The listing builds one solid part. Answer for the finished solid, in the listing's coordinates (mm). Face numbers are marked on the shaded views. A direction names the side the tool comes from. Coordinates: 2 decimals unless noted, no trailing zeros. Loops run counter-clockwise (first coordinate to the right, second up) from the corner with the lowest first, then second, coordinate; pieces in that order, holes last. Notation, with made-up numbers: (1.25, 14.5) -> (29.25, 14.5) arc R16 cw to (29.25, 32.5) -> close; hole circle Ø8 at (-12, 1). An arc over 180 degrees is marked (long way). Answer in a Markdown table with one row per item.
```python
from build123d import *

# Parameters (mm, degrees)
BOSS_EXTRUDE1_DEPTH = 34
SKETCH2_W           = 6.25
SKETCH2_H           = 31.7
CUT_EXTRUDE1_DEPTH  = 12
SKETCH3_W           = 10
SKETCH3_H           = 25
CUT_EXTRUDE2_DEPTH  = 12
SKETCH4_W           = 6
SKETCH4_H           = 10
CUT_EXTRUDE3_DEPTH  = 10
CHAMFER2_SIZE       = 1.5
CHAMFER3_SIZE       = 1.5
CHAMFER4_SIZE       = 1.5
CHAMFER4_SIZE_2     = 4.815472512


with BuildPart() as part:
    # Sketch1 → Boss-Extrude1 (new body)
    with BuildSketch(Plane(origin=(0, 0, 0), x_dir=(1, 0, 0), z_dir=(0, 1, 0))):
        Polygon((6.5, 4.75), (12.5, 4.75), (6.5, -4.75), (-6.5, -4.75), (-6.5, 4.75), align=None)
    extrude(amount=BOSS_EXTRUDE1_DEPTH)

    # Sketch2 → Cut-Extrude1 (cut)
    with BuildSketch(Plane.ZY.offset(6.5)):
        with Locations((0, 17)):
            Rectangle(SKETCH2_W, SKETCH2_H)
    extrude(amount=-CUT_EXTRUDE1_DEPTH, mode=Mode.SUBTRACT)

    # Sketch3 → Cut-Extrude2 (cut)
    with BuildSketch(Plane.XY.offset(4.75)):
        with Locations((-1.5, 17)):
            Rectangle(SKETCH3_W, SKETCH3_H)
    extrude(amount=-CUT_EXTRUDE2_DEPTH, mode=Mode.SUBTRACT)

    # Sketch4 → Cut-Extrude3 (cut)
    with BuildSketch(Plane.XY.offset(4.75)):
        with Locations((9.5, 29)):
            Rectangle(SKETCH4_W, SKETCH4_H)
        with Locations((9.5, 5)):
            Rectangle(SKETCH4_W, SKETCH4_H)
    extrude(amount=-CUT_EXTRUDE3_DEPTH, mode=Mode.SUBTRACT)

    # Chamfer2
    chamfer2_edges = [part.edges().sort_by_distance(p)[0] for p in [
        (6.5, 29, 4.75),
    ]]
    chamfer(chamfer2_edges, length=CHAMFER2_SIZE)

    # Chamfer3
    chamfer3_edges = [part.edges().sort_by_distance(p)[0] for p in [
        (6.5, 5, 4.75),
    ]]
    chamfer(chamfer3_edges, length=CHAMFER3_SIZE)

    # Chamfer4
    # the kernel refuses this chamfer: 4.815472512, 1.5 mm, written as the material it takes off along each edge
    with BuildSketch(Plane(origin=(6.5, -2.508851902, 4.75), x_dir=(-0.9965532165776719, 0, 0.08295593124482357), z_dir=(0, 1, 0))) as chamfer4_piece_1:
        Polygon((CHAMFER4_SIZE * 0.996553216578, -CHAMFER4_SIZE * 0.0829559312448), (-CHAMFER4_SIZE_2 * 0.602290752459, -CHAMFER4_SIZE_2 * 0.798276799955), (0, 0), align=None)
    extrude(amount=39.017703804, mode=Mode.SUBTRACT)


solid = part.part
```
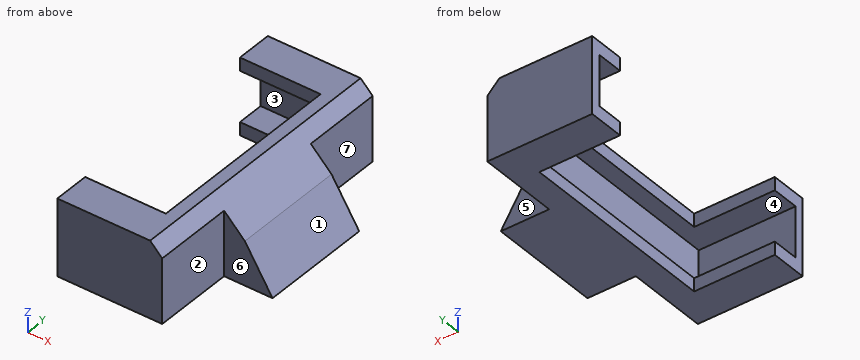
Item 1: Find the intervals of material crossed by probe 1 along Y at (x, z) = (0.75, -1.25); probe 2 along Z at (x, y) = (0.25, 31) (3 decimals); probe 3 along X at (y, z) = (9, 0.5), in increasing order.
Findings below:
| item | result |
|---|---|
| probe 1 | y = 0 to 1.15, 32.85 to 34 |
| probe 2 | z = -4.75 to -3.125, 3.125 to 4.75 |
| probe 3 | x = 5.5 to 6.5 |
Item 2: A cutting plane is placed at B-B, the plane y = 8. Determine the outline of the cut face in (x, z) (3 decimals), plus the area to 3 significant figures.
Findings below:
| item | result |
|---|---|
| outline | (3.5, -4.75) -> (6.5, -4.75) -> (6.5, 3.25) -> (5, 4.75) -> (3.5, 4.75) -> (3.5, 3.125) -> (5.5, 3.125) -> (5.5, -3.125) -> (3.5, -3.125) -> close |
| area | 14.9 mm2 |
Item 3: A tool of negligible diameter and unlimited length cuts with its end or side. For the marked faces 1, 2 and 3, from which of +Z, -Z, +X, -X, +Y, -Y can it reach the whole face along a straight path? Write none if from no direction.
Findings below:
| item | result |
|---|---|
| face 1 | +Z, +X, +Y, -Y |
| face 2 | +Z, -Z, +X, -Y |
| face 3 | -X |
Item 4: A cutting plane is placed at D-D, the plane x = 0.25. Determine the outline of the cut face in (y, z) (3 decimals), plus the area to 3 significant figures.
Findings below:
| item | result |
|---|---|
| outline | (0, -4.75) -> (4.5, -4.75) -> (4.5, -3.125) -> (1.15, -3.125) -> (1.15, 3.125) -> (4.5, 3.125) -> (4.5, 4.75) -> (0, 4.75) -> close; (29.5, -4.75) -> (34, -4.75) -> (34, 4.75) -> (29.5, 4.75) -> (29.5, 3.125) -> (32.85, 3.125) -> (32.85, -3.125) -> (29.5, -3.125) -> close |
| area | 43.6 mm2 |
Item 5: A cutting plane is placed at A-A, the plane x = 4.5. Determine the outline of the cut face in (y, z) (3 decimals).
Findings below:
| item | result |
|---|---|
| outline | (0, -4.75) -> (34, -4.75) -> (34, 4.75) -> (0, 4.75) -> close; hole (1.15, -3.125) -> (32.85, -3.125) -> (32.85, 3.125) -> (1.15, 3.125) -> close |
Item 6: Determine the mould class of the marked faces 4, 5, 6 and 7 for opening direction Y: +Y half, -Y half, draft (parallel to the pull), parting line (faces both ways), or undercut.
Findings below:
| item | result |
|---|---|
| face 4 | undercut |
| face 5 | +Y half |
| face 6 | -Y half |
| face 7 | draft |
Item 7: A cutting plane is placed at C-C, the plane z = 1.75. Determine the outline of the cut face in (x, y), plus the area to 3 significant figures.
Findings below:
| item | result |
|---|---|
| outline | (-6.5, 0) -> (6.5, 0) -> (6.5, 10) -> (8, 10) -> (8, 24) -> (6.5, 24) -> (6.5, 34) -> (-6.5, 34) -> (-6.5, 32.85) -> (5.5, 32.85) -> (5.5, 1.15) -> (-6.5, 1.15) -> close |
| area | 82.6 mm2 |
Item 8: Flat-ended cylindrical pins translate along their axes: pin 1 Ø3 at (x, z) = (11, -2) entering from +Y; pin 2 Ø1.3 at (y, z) = (20, 4) entering from -X; pin 3 Ø5 at (y, z) = (19, -0.5) entering from -X. Find the tip coordinate at first contact, or state that the pin passes through.
Findings below:
| item | result |
|---|---|
| pin 1 | stops at y = 24 |
| pin 2 | stops at x = 3.5 |
| pin 3 | stops at x = 5.5 |
